Can you work these out from the drawing? Everything is in mm from the part's minimum corner. Give positions to 0.01 mm unless a question says otherwise; leave off trailing zeros. Order: outer loops, then holes, each group sorted by start corner. A loop starts at its lowest first (then second) coordinate and runs counter-clockwise, first axis right, second up. Notation, with made-up numbers: (-11.75, 39.5) -> (-7.75, 39.5) arc R21 cw to (-7.75, 65.5) -> close; hole circle Ø7 at (6, 40.25). An arc over 180 degrees is marked (long way). One line per item, written item: value.
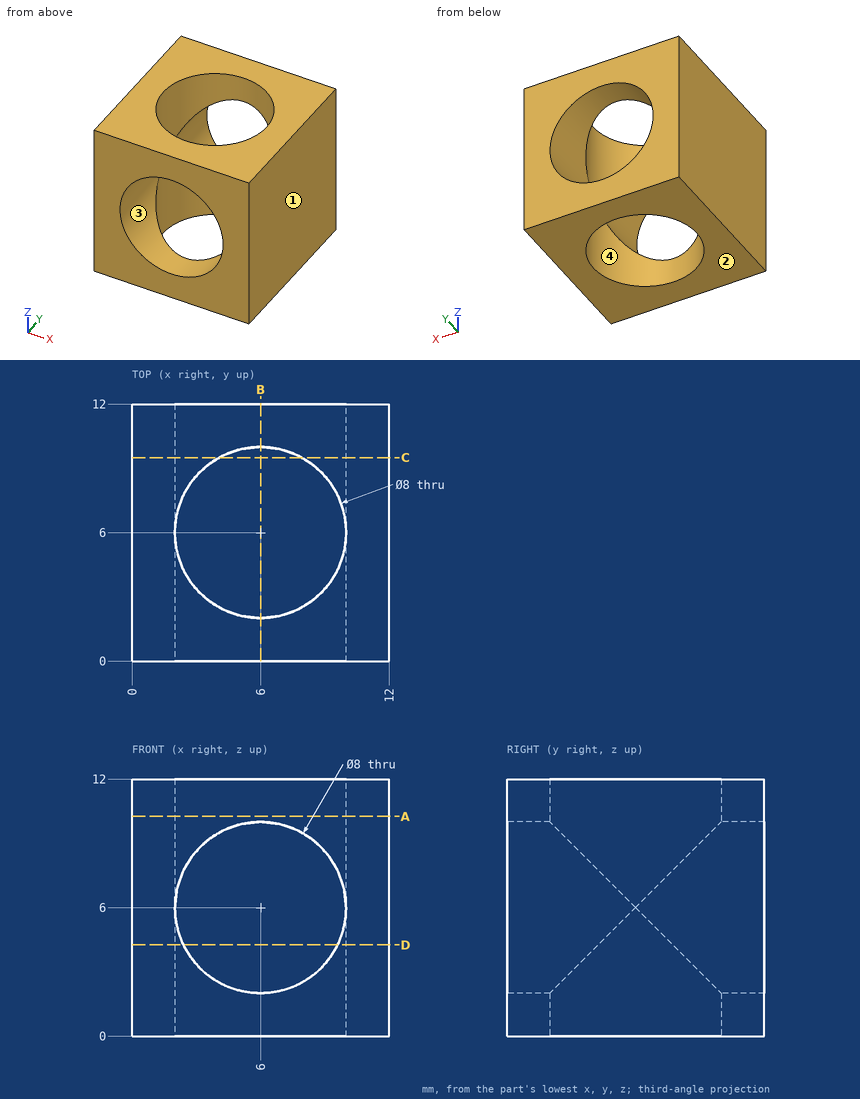
1) We'd pull the mould along X, two halves only. Please class the marked faces 1, 2, 3 and 4: +X half, -X half, draft (parallel to the pull), parting line (faces both ways), or undercut.
Answer below:
face 1: +X half
face 2: draft
face 3: undercut
face 4: undercut
2) If I drill on line 1 along X through (y, z) = (1.5, 6); line 2 along X through (y, z) = (7.5, 9.75); line 3 along Y through (x, z) = (5.75, 11.5), over which ranges is the centre line in solid material (lowest first)?
Answer below:
line 1: x = 0 to 2, 10 to 12
line 2: x = 0 to 2.29, 9.71 to 12
line 3: y = 0 to 2.01, 9.99 to 12
3) Suppose I cut it at B-B, the plane x = 6. Write out the boundary of the cut face in (y, z).
Answer below:
outline: (0, 0) -> (2, 0) -> (2, 2) -> (0, 2) -> close; (0, 10) -> (2, 10) -> (2, 12) -> (0, 12) -> close; (10, 0) -> (12, 0) -> (12, 2) -> (10, 2) -> close; (10, 10) -> (12, 10) -> (12, 12) -> (10, 12) -> close
4) Suppose I cut it at D-D, the plane z = 4.25. Write out the boundary of the cut face in (x, y).
Answer below:
outline: (0, 0) -> (2.4, 0) -> (2.4, 4.25) arc R4 cw to (2.4, 7.75) -> (2.4, 12) -> (0, 12) -> close; (9.6, 0) -> (12, 0) -> (12, 12) -> (9.6, 12) -> (9.6, 7.75) arc R4 cw to (9.6, 4.25) -> close
5) Suppose I cut it at A-A, the plane z = 10.25. Write out the boundary of the cut face in (x, y), then the cut area to 3 significant figures.
Answer below:
outline: (0, 0) -> (12, 0) -> (12, 12) -> (0, 12) -> close; hole circle Ø8 at (6, 6)
area: 93.7 mm2
6) Suppose I cut it at C-C, the plane y = 9.5. Write out the boundary of the cut face in (x, z).
Answer below:
outline: (0, 0) -> (4.06, 0) -> (4.06, 2.5) arc R4 cw to (4.06, 9.5) -> (4.06, 12) -> (0, 12) -> close; (7.94, 0) -> (12, 0) -> (12, 12) -> (7.94, 12) -> (7.94, 9.5) arc R4 cw to (7.94, 2.5) -> close
